from build123d import *

# Parameters (mm, degrees)
SKETCH1_W                = 200
SKETCH1_H                = 213
BOSS_EXTRUDE1_DEPTH      = 12.5
FILLET1_R                = 10
BOSS_EXTRUDE2_DEPTH      = 70
BOSS_EXTRUDE3_DEPTH      = 10
CUT_EXTRUDE1_DEPTH       = 20
SKETCH5_R                = 7.5
CUT_EXTRUDE2_DEPTH       = 20
SKETCH6_R                = 15
CUT_EXTRUDE3_DEPTH       = 10
SKETCH8_R                = 35
BOSS_EXTRUDE4_DEPTH      = 10
BOSS_EXTRUDE4_DEPTH_BACK = 120
SKETCH9_R                = 20.5
CUT_EXTRUDE4_DEPTH       = 224
SKETCH10_R               = 41.5
SKETCH10_R_2             = 20.5
BOSS_EXTRUDE5_DEPTH      = 10
BOSS_EXTRUDE5_DEPTH_BACK = 120
SKETCH11_R               = 20.5
CUT_EXTRUDE5_DEPTH       = 201


with BuildPart() as part:
    # Sketch1 → Boss-Extrude1 (new body, symmetric)
    with BuildSketch(Plane(origin=(0, 0, 0), x_dir=(1, 0, 0), z_dir=(0, 1, 0))):
        Rectangle(SKETCH1_W, SKETCH1_H)
    extrude(amount=BOSS_EXTRUDE1_DEPTH, both=True)

    # Fillet1
    fillet1_edges = [part.edges().sort_by_distance(p)[0] for p in [
        (100, 0, 106.5),
        (-100, 0, 106.5),
        (-100, 0, -106.5),
        (100, 0, -106.5),
    ]]
    fillet(fillet1_edges, radius=FILLET1_R)

    # Sketch2 → Boss-Extrude2 (add)
    with BuildSketch(Plane(origin=(0, 12.5, 0), x_dir=(1, 0, 0), z_dir=(0, 1, 0))):
        with BuildLine():
            Line((-70, -106.5), (-55, -106.5))
            Line((-55, -106.5), (-55, -38.928392203))
            ThreePointArc((-55, -38.928392203), (0.920301962, -7.420301962), (32.428392203, 48.5))
            Line((32.428392203, 48.5), (100, 48.5))
            Line((100, 48.5), (100, 63.5))
            Line((100, 63.5), (20, 63.5))
            ThreePointArc((20, 63.5), (-9.686299755, 3.186299755), (-70, -26.5))
            Line((-70, -26.5), (-70, -106.5))
        make_face()
    extrude(amount=BOSS_EXTRUDE2_DEPTH)

    # Sketch3 → Boss-Extrude3 (add)
    with BuildSketch(Plane(origin=(0, 12.5, 0), x_dir=(1, 0, 0), z_dir=(0, 1, 0))):
        with BuildLine():
            Line((100, -46.5), (55, -46.5))
            ThreePointArc((55, -46.5), (44.393398282, -50.893398282), (40, -61.5))
            Line((40, -61.5), (40, -106.5))
            Line((40, -106.5), (90, -106.5))
            ThreePointArc((90, -106.5), (97.071067812, -103.571067812), (100, -96.5))
            Line((100, -96.5), (100, -46.5))
        make_face()
    extrude(amount=BOSS_EXTRUDE3_DEPTH)

    # Sketch4 → Cut-Extrude1 (cut)
    with BuildSketch(Plane(origin=(0, 12.5, 0), x_dir=(1, 0, 0), z_dir=(0, 1, 0))):
        with BuildLine():
            Line((-46, -97.5), (-46, -45.782855831))
            ThreePointArc((-46, -45.782855831), (7.284262993, -13.784262993), (39.282855831, 39.5))
            Line((39.282855831, 39.5), (91, 39.5))
            Line((91, 39.5), (91, -37.5))
            Line((91, -37.5), (55, -37.5))
            ThreePointArc((55, -37.5), (38.029437252, -44.529437252), (31, -61.5))
            Line((31, -61.5), (31, -87.5))
            ThreePointArc((31, -87.5), (28.071067812, -94.571067812), (21, -97.5))
            Line((21, -97.5), (-46, -97.5))
        make_face()
    extrude(amount=-CUT_EXTRUDE1_DEPTH, mode=Mode.SUBTRACT)

    # Sketch5 → Cut-Extrude2 (cut)
    with BuildSketch(Plane(origin=(0, 22.5, 0), x_dir=(1, 0, 0), z_dir=(0, 1, 0))):
        with Locations((70.732233047, -77.232233047)):
            Circle(SKETCH5_R)
    extrude(amount=-CUT_EXTRUDE2_DEPTH, mode=Mode.SUBTRACT)

    # Sketch6 → Cut-Extrude3 (cut)
    with BuildSketch(Plane(origin=(0, 22.5, 0), x_dir=(1, 0, 0), z_dir=(0, 1, 0))):
        with Locations((70.732233047, -77.232233047)):
            Circle(SKETCH6_R)
    extrude(amount=-CUT_EXTRUDE3_DEPTH, mode=Mode.SUBTRACT)

    # Sketch8 → Boss-Extrude4 (add, two sides)
    with BuildSketch(Plane.XY.offset(106.5)) as boss_extrude4_sk:
        with Locations((-62.5, 82.5)):
            Circle(SKETCH8_R)
    extrude(amount=BOSS_EXTRUDE4_DEPTH)
    extrude(boss_extrude4_sk.sketch, amount=-BOSS_EXTRUDE4_DEPTH_BACK)

    # Sketch9 → Cut-Extrude4 (cut, through all)
    with BuildSketch(Plane.XY.offset(116.5)):
        with Locations((-62.5, 82.5)):
            Circle(SKETCH9_R)
    extrude(amount=-CUT_EXTRUDE4_DEPTH, mode=Mode.SUBTRACT)

    # Sketch10 → Boss-Extrude5 (add, two sides)
    with BuildSketch(Plane(origin=(100, 0, 0), x_dir=(0, 0, -1), z_dir=(1, 0, 0))) as boss_extrude5_sk:
        with Locations((56, 82.5)):
            Circle(SKETCH10_R)
        with Locations((56, 82.5)):
            Circle(SKETCH10_R_2, mode=Mode.SUBTRACT)
    extrude(amount=BOSS_EXTRUDE5_DEPTH)
    extrude(boss_extrude5_sk.sketch, amount=-BOSS_EXTRUDE5_DEPTH_BACK)

    # Sketch11 → Cut-Extrude5 (cut, through all)
    with BuildSketch(Plane(origin=(100, 0, 0), x_dir=(0, 0, -1), z_dir=(1, 0, 0))):
        with Locations((56, 82.5)):
            Circle(SKETCH11_R)
    extrude(amount=-CUT_EXTRUDE5_DEPTH, mode=Mode.SUBTRACT)


solid = part.part
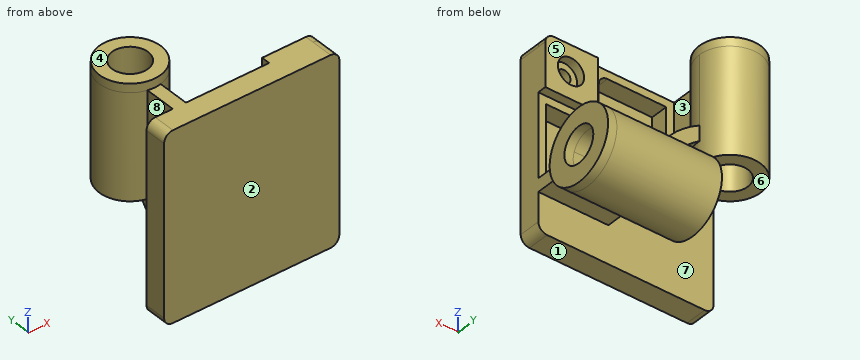
Can you work these out from the model? Positions are in its coordinate system, mm. Face numbers are marked on the shaded views. A direction names the side the tool comes from. Round coordinates to 2 decimals unless told otherwise and drop trailing zeros. Write each loop counter-clockwise with the first axis right and the second up, starting at its lowest first coordinate (ties: lowest second). Pieces come first, ordered by that corner, then holes. Notation, with made-up numbers: M 70.25,-9.5 L 90.25,-9.5 A9 ccw 90.25,2.5 Z; hole C 48,69 d11. An arc over 180 degrees is marked long. Use a Markdown table: item, result.
Item 1: I want a section at A-A (z = 8). List the corners of the cut face in (x, y) for me, and give its area (3 significant figures).
Found:
| item | result |
|---|---|
| outline | M -100,-12.5 L 100,-12.5 L 100,12.5 L 91,12.5 L 91,-7.5 L 12.72,-7.5 L 12.72,12.5 L 0.34,12.5 L 0.34,82.5 L -22.9,82.5 L -22.9,12.5 L -100,12.5 Z; C -62.5,82.5 d70; hole C -62.5,82.5 d41 |
| area | 7,590 mm2 |
Item 2: We'd pull the mould along Y, two halves only. Please class the marked faces 1, 2 and 3: released by +Y, released by -Y, zero draft, split by the parting line, or undercut.
Found:
| item | result |
|---|---|
| face 1 | zero draft |
| face 2 | released by -Y |
| face 3 | undercut |
Item 3: I want a section at B-B (z = 102.5). List the corners of the cut face in (x, y) for me, and give its area (3 significant figures).
Found:
| item | result |
|---|---|
| outline | M -98,-12.5 L 98,-12.5 L 98,22.5 L 40,22.5 L 40,12.5 L -55,12.5 L -55,48.31 A35 ccw long -70,48.31 L -70,12.5 L -98,12.5 Z; hole C -62.5,82.5 d41 |
| area | 8,540 mm2 |
Item 4: For pin 1 Ø2 at (x, y) = (53.5, 99.5) entering from -Z; pin 2 Ø3 at (y, z) = (18.5, 82.5) entering from -X; pin 3 Ø10 at (x, y) = (67, 1) entering from +Z, each with a flat end and sliding along its axis, tell me the tip position at first contact or that it passes through.
Found:
| item | result |
|---|---|
| pin 1 | stops at z = -94.29 |
| pin 2 | stops at x = -70 |
| pin 3 | stops at z = 106.5 |
Item 5: If I drill on line 1 along X through (y, z) = (0, 76.5); line 2 along X through (y, z) = (83, 99.5); line 3 along Y through (x, z) = (68, -56), over which ranges is the centre line in solid material (lowest first)? Write a range as [from, to].
Found:
| item | result |
|---|---|
| line 1 | x = [-100, -46], [31, 100] |
| line 2 | x = [-97.5, -82.99], [-42.01, -27.5] |
| line 3 | y = [-12.5, 62], [103, 124] |
Item 6: I want a section at D-D (x = 49). List the corners of the cut face in (y, z) for me, and give its area (3 significant figures).
Found:
| item | result |
|---|---|
| outline | M -12.5,-106.5 L 12.5,-106.5 L 12.5,-63.5 L 41.68,-63.5 A41.5 ccw long 41.68,-48.5 L 12.5,-48.5 L 12.5,-39.5 L -7.5,-39.5 L -7.5,38.26 L 12.5,38.26 L 12.5,47.75 L 22.5,47.75 L 22.5,106.5 L -12.5,106.5 Z; hole C 82.5,-56 d41 |
| area | 8,880 mm2 |
Item 7: Which directions (+Z, -Z, +X, -X, +Y, -Y) give clear straight access to the entire face, cutting with the end or side of a thin tool? Please do the marked faces 4, 5, 6, 7 and 8.
Found:
| item | result |
|---|---|
| face 4 | +Z, +X, -X, +Y, -Y |
| face 5 | +Z, +X, +Y |
| face 6 | -Z, -X, +Y |
| face 7 | -Z, -X |
| face 8 | +Z, -Z, -X |
Item 8: I want a section at C-C (x = -62.5). List the corners of the cut face in (y, z) for me, and give its area (3 significant figures).
Found:
| item | result |
|---|---|
| outline | M -12.5,-106.5 L 12.5,-106.5 L 12.5,25.24 L 47.5,25.24 L 47.5,-13.5 L 62,-13.5 L 62,116.5 L 47.5,116.5 L 47.5,106.5 L -12.5,106.5 Z; M 103,-13.5 L 117.5,-13.5 L 117.5,116.5 L 103,116.5 Z |
| area | 11,900 mm2 |
